The drawing under review shows one solid part. Ordinate dimensions are in mm from its lowest x, y, z. A direction names the side the tool comes from. Give positions to 0.01 mm unless a question says otherwise; leave off trailing zeros. Order: outer loops, then holes, each group sorted by start corner. A loop starts at its lowest first (then second) coordinate and runs counter-clockwise, first axis right, second up. Notation, with made-up numbers: M 24,-33 L 46,-33 A24 ccw 46,-4 Z; hole C 19,26 d6. An arc over 180 degrees is marked long. Put each result on its own line as item: value. Start each with the question number.
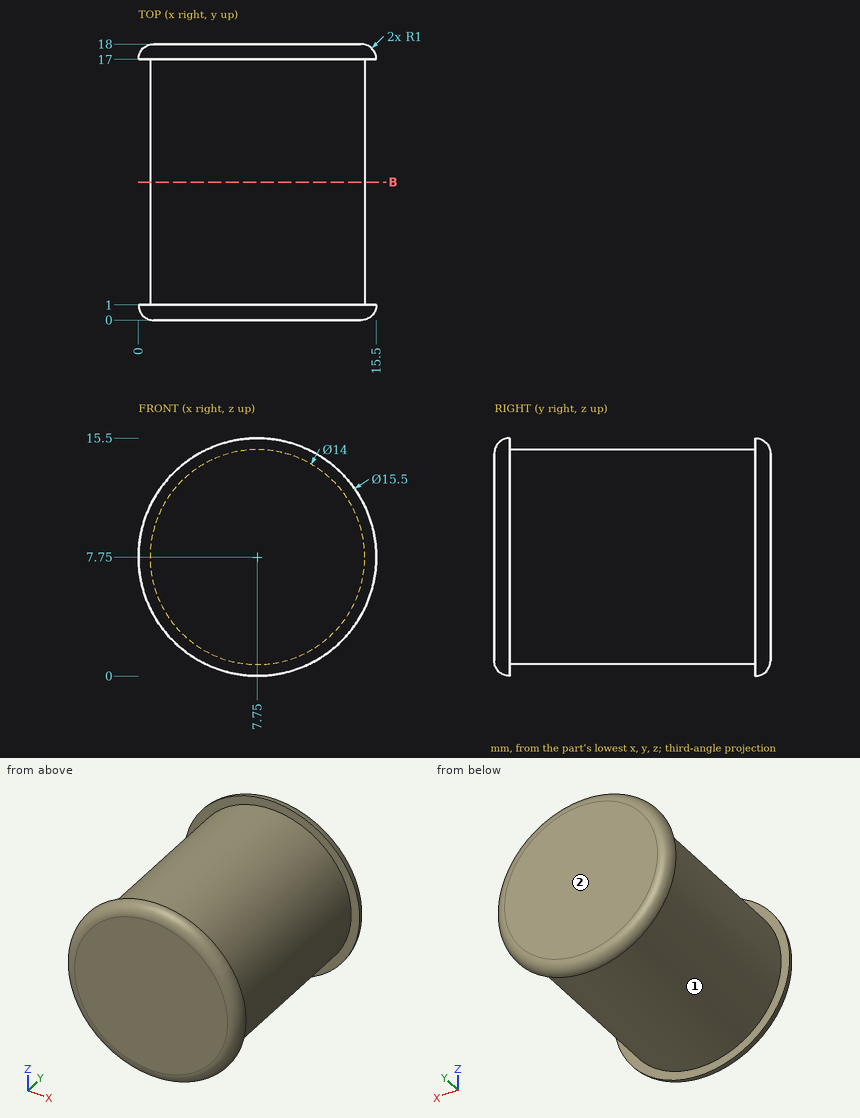
1. Machinability: for the marked faces 1 and 2, which of the approach directions +Z, -Z, +X, -X, +Y, -Y give a long, thin tool a straight path to every point of the face, cutting with its end or side? Answer none if there is none.
2. To check wall thickness, follow probe 1 along Z at (x, y) = (7.5, 11); probe 2 along X at (y, z) = (7.25, 2); probe 3 along X at (y, z) = (10.25, 12.25). State the ranges of each line that lie inside material, in increasing order.
3. Insertion check: pin 1 (3 mm diameter, centred on x = 12, y = 6, fed in from +Z); pin 2 (8 mm diameter, centred on y = 7, z = 12, fed in from +X); pin 3 (3 mm diameter, centred on y = 12, z = 2.5, fed in from +X). Each pin has a flat end and moves straight along its axis. Give the tip position at first contact, or say it passes through.
4. Consider section B-B on y = 9. Give the boundary of the cut face in (x, z), then the cut area to 3 significant figures.
Returned:
1. face 1: none
1. face 2: +Z, -Z, +X, -X, +Y
2. probe 1: z = 0.75 to 14.75
2. probe 2: x = 3.76 to 11.74
2. probe 3: x = 2.39 to 13.11
3. pin 1: stops at z = 14.19
3. pin 2: stops at x = 14.75
3. pin 3: stops at x = 13.66
4. outline: C 7.75,7.75 d14
4. area: 154 mm2
